Can you work these out from the model? Positions are in its coordinate system, mm. Give positions to 0.01 mm unless a question says otherwise; leave off trailing zeros. Loops run counter-clockwise (first coordinate to the right, second up) from the corner with the lowest first, then second, coordinate; pieces in that order, holes last. Notation, with made-up numbers: M 58,-18 L 102,-18 A25 ccw 102,8 Z; hole C -30,72.25 d6. An arc over 180 degrees is marked long. Use CSV: the item, a comma, the result in double quotes.
from build123d import *

# Parameters (mm, degrees)
SWEEP1_PROFILE_R    = 3.175
SWEEP2_PROFILE_R    = 3.175
SKETCH42_W          = 31.75
SKETCH42_H          = 285.7
BOSS_EXTRUDE1_DEPTH = 3.81


with BuildPart() as part:
    # Sweep1: sweep along a path in Sketch1
    with BuildLine(Plane.XY) as sweep1_path:
        Line((0, 0), (0, 114.3))
    # Sweep1 profile (on start of the path) → Sweep1 (sweep)
    with BuildSketch(Plane.ZX):
        Circle(SWEEP1_PROFILE_R)
    sweep(path=sweep1_path.line)



with BuildPart() as body_2:
    # Sweep2: sweep along a path in Sketch1<3>
    with BuildLine(Plane.XY) as sweep2_path:
        Line((25.4, 114.3), (25.4, 0))
    # Sweep2 profile (on start of the path) → Sweep2 (sweep)
    with BuildSketch(Plane(origin=(25.4, 114.3, 0), x_dir=(-1, 0, 0), z_dir=(0, -1, 0))):
        Circle(SWEEP2_PROFILE_R)
    sweep(path=sweep2_path.line)


with BuildPart() as part_1:
    add(part.part)

    add(body_2.part)  # Boss-Extrude1 merges body 2
    # Sketch42 → Boss-Extrude1 (add, symmetric)
    with BuildSketch(Plane.XY):
        with Locations((12.7, 257.15)):
            Rectangle(SKETCH42_W, SKETCH42_H)
    extrude(amount=BOSS_EXTRUDE1_DEPTH, both=True)


solid = part_1.part
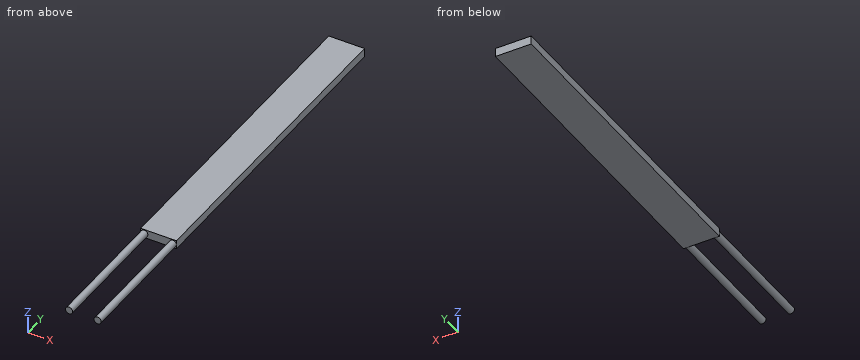
Q1. I want a section at C-C, the plane x = 16. Please give me the cut outline in (y, z), then the cut area to 3 significant figures.
Model answer:
outline,"M 114.3,-3.81 L 400,-3.81 L 400,3.81 L 114.3,3.81 Z"
area,"2,180 mm2"
Q2. Please list where this line runs through material, in increasing order: L1, parallel to Y at x = 14, z = -0.75. Write a range as from..to.
Model answer:
L1,"114.3..400"
Q3. I want a section at B-B, the plane z = -1.5. Please give me the cut outline in (x, y) (3 decimals).
Model answer:
outline,"M -3.175,114.3 L -2.798,114.3 L -2.798,0 L 2.798,0 L 2.798,114.3 L 22.602,114.3 L 22.602,0 L 28.198,0 L 28.198,114.3 L 28.575,114.3 L 28.575,400 L -3.175,400 Z"
Q4. I want a section at A-A, the plane y = 106.5. Please give me the cut outline in (x, z) (3 decimals), then the cut area to 3 significant figures.
Model answer:
outline,"C 0,0 d6.35; C 25.4,0 d6.35"
area,"63.3 mm2"
Q5. I'm going to push flat-ended pins straight in: P1, Ø6, axis at x = 17, y = 63, coming from the +Z side; P2, Ø2.5, axis at x = 5.5, z = -1, coming from the -Y side. Where does each tip first touch, or does it pass through?
Model answer:
P1,"through"
P2,"y = 114.3"
